For this review, take the finished solid that the model builds, in its own axes (mm). A direction names the side the tool comes from. Round coordinates to 2 decimals unless told otherwise and drop trailing zeros. Write each loop counter-clockwise with the first axis right and the second up, starting at its lowest first coordinate (ties: lowest second). Pieces come first, ordered by that corner, then holes. Notation, with made-up numbers: (11.25, -25.5) - (22.25, -25.5) arc R28 cw to (22.25, 0.5) - close; hole circle Ø5 at (-0.75, -12). An arc over 180 degrees is marked (long way). Answer in a Markdown table with one row per item. Add a question column.
from build123d import *

# Parameters (mm, degrees)
SKETCH1_W           = 10
SKETCH1_H           = 12.1
BOSS_EXTRUDE1_DEPTH = 30
SKETCH2_R           = 2
BOSS_EXTRUDE2_DEPTH = 0.7
BOSS_EXTRUDE3_DEPTH = 9.3
FILLET1_R           = 1
SKETCH4_W           = 12.1
SKETCH4_H           = 6
BOSS_EXTRUDE4_DEPTH = 14


with BuildPart() as part:
    # Sketch1 → Boss-Extrude1 (new body)
    with BuildSketch(Plane(origin=(0, 0, 0), x_dir=(1, 0, 0), z_dir=(0, 1, 0))):
        Rectangle(SKETCH1_W, SKETCH1_H)
    extrude(amount=BOSS_EXTRUDE1_DEPTH)

    # Sketch2 → Boss-Extrude2 (add)
    with BuildSketch(Plane(origin=(0, 30, 0), x_dir=(1, 0, 0), z_dir=(0, 1, 0))):
        with Locations(Location((0, 0, 0), (0, 0, 270))):
            Circle(SKETCH2_R)
    extrude(amount=BOSS_EXTRUDE2_DEPTH)

    # Sketch3 → Boss-Extrude3 (add)
    with BuildSketch(Plane(origin=(0, 30.7, 0), x_dir=(1, 0, 0), z_dir=(0, 1, 0))):
        with BuildLine():
            ThreePointArc((1.5, 0), (1.08976923, 1.030729365), (0.083462634, 1.497676196))
            Line((0.083462634, 1.497676196), (-1.497676196, -0.083462634))
            ThreePointArc((-1.497676196, -0.083462634), (0.041747489, -1.499418937), (1.5, 0))
        make_face()
    extrude(amount=BOSS_EXTRUDE3_DEPTH)

    # Fillet1
    fillet1_edges = [part.edges().sort_by_distance(p)[0] for p in [
        (5, 15, 6.05),
        (-5, 15, 6.05),
        (-5, 15, -6.05),
        (5, 15, -6.05),
    ]]
    fillet(fillet1_edges, radius=FILLET1_R)

    # Sketch4 → Boss-Extrude4 (add)
    with BuildSketch(Plane(origin=(0, 0, 0), x_dir=(0, 0, -1), z_dir=(1, 0, 0))):
        with Locations((0, 3)):
            Rectangle(SKETCH4_W, SKETCH4_H)
    extrude(amount=BOSS_EXTRUDE4_DEPTH)


solid = part.part
Q1. Insertion check: pin 1 Ø3 at (x, z) = (-2.5, -2.5) entering from +Y; pin 2 Ø2 at (y, z) = (19, 2) entering from +X; pin 3 Ø2 at (x, z) = (9.5, -2.5) entering from +Y; pin 4 Ø4 at (x, z) = (9.5, 1.5) entering from -Y. Each pin has a flat end and moves straight along its axis. Give the tip position at first contact, or say it passes through.
Q2. Add section D-D on y = 35.5. State the section outline as (x, z) points.
Q3. Add section C-C on x = 5.75. State the section outline as (y, z) points.
Q4. Tool access review of faces 1 (the face through (5, 18, 0)), 2 (the face through (-1, 30.7, -1)), 3 (the face through (4.699, 18.168, -5.765)), 4 (the face through (-0.696, 35.285, -0.718)): name each direction out of +Z, -Z, +X, -X, +Y, -Y from which nothing blocks a thin tool from reaching the whole face with its end or side.
Q5. Add section A-A on z = -4.5. State the section outline as (x, y) points.
Q6. Add section B-B on y = 18. State the section outline as (x, z) points, then the cut area to 3 significant figures.
Q7. To check wall thickness, follow probe 1 along Y at (x, z) = (9.25, 5); probe 2 along X at (y, z) = (14.5, 2.75); probe 3 along Y at (x, z) = (4.5, 4.75). State the ranges of each line that lie inside material, in increasing order.
Answer sheet:
| question | item | result |
|---|---|---|
| 1 | pin 1 | stops at y = 30 |
| 1 | pin 2 | stops at x = 5 |
| 1 | pin 3 | stops at y = 6 |
| 1 | pin 4 | stops at y = 0 |
| 2 | outline | (-1.5, 0.08) - (0.08, -1.5) arc R1.5 ccw (long way) to start |
| 3 | outline | (0, -6.05) - (6, -6.05) - (6, 6.05) - (0, 6.05) - close |
| 4 | face 1 | +Z, -Z, +X, +Y |
| 4 | face 2 | +Y |
| 4 | face 3 | -Z, +X, +Y |
| 4 | face 4 | -Z, -X, +Y |
| 5 | outline | (-5, 0) - (14, 0) - (14, 6) - (5, 6) - (5, 30) - (-5, 30) - close |
| 6 | outline | (-5, -5.05) arc R1 ccw to (-4, -6.05) - (4, -6.05) arc R1 ccw to (5, -5.05) - (5, 5.05) arc R1 ccw to (4, 6.05) - (-4, 6.05) arc R1 ccw to (-5, 5.05) - close |
| 6 | area | 120 mm² |
| 7 | probe 1 | y = 0 to 6 |
| 7 | probe 2 | x = -5 to 5 |
| 7 | probe 3 | y = 0 to 30 |
